Geometry check sheet. Reference: the model listing, model coordinates, mm. Face numbers are marked on the shaded views. Coordinates: 2 decimals unless noted, no trailing zeros. Loops run counter-clockwise (first coordinate to the right, second up) from the corner with the lowest first, then second, coordinate; pieces in that order, holes last.
from build123d import *

# Parameters (mm, degrees)
SKETCH2_R                = 0.85
CUT_EXTRUDE1_DEPTH       = 2.54
BOSS_EXTRUDE1_DEPTH      = 12.7
BOSS_EXTRUDE1_DEPTH_BACK = 2.54
SKETCH3_R                = 1.9
SKETCH4_R                = 0.85
CUT_EXTRUDE2_DEPTH       = 2.794


with BuildPart() as part:
    # Sketch1 → Revolve1 (revolve)
    with BuildSketch(Plane.XY, mode=Mode.PRIVATE) as revolve1_sk:
        Polygon((0, 0), (0, 8.5), (5.21775571, 8.5), (5.21775571, 8), (5.71775571, 8), (5.71775571, 8.5), (11.139308543, 8.5), (11.139308543, 8), (11.639308543, 8), (11.639308543, 8.5), (14.5, 8.5), (14.5, 0), align=None)
    revolve(revolve1_sk.sketch.rotate(Axis((0, 0, 0), (1, 0, 0)), 90), axis=Axis((0, 0, 0), (1, 0, 0)))

    # Sketch2 → Cut-Extrude1 (cut)
    with BuildSketch(Plane.ZY):
        with Locations((-2.641364136, 5.664423669)):
            Circle(SKETCH2_R)
        with Locations((6.226216863, -0.544723392)):
            Circle(SKETCH2_R)
        with Locations((-3.584852727, -5.119700277)):
            Circle(SKETCH2_R)
    extrude(amount=-CUT_EXTRUDE1_DEPTH, mode=Mode.SUBTRACT)

    # Sketch3 → Boss-Extrude1 (add, two sides: drawn at the far end of the back side and taken through both)
    with BuildSketch(Plane(origin=(0, -7.361215932, 4.25), x_dir=(1, 0, 0), z_dir=(0, -0.8660254037844398, 0.499999999999998)).offset(-BOSS_EXTRUDE1_DEPTH_BACK)):
        with Locations(Location((2.694505782, 0, 0), (0, 0, 270))):
            Circle(SKETCH3_R)
    extrude(amount=BOSS_EXTRUDE1_DEPTH + BOSS_EXTRUDE1_DEPTH_BACK)

    # Sketch4 → Cut-Extrude2 (cut)
    with BuildSketch(Plane(origin=(14.5, 0, 0), x_dir=(0, 0, -1), z_dir=(1, 0, 0))):
        with Locations((0, -6.25)):
            Circle(SKETCH4_R)
        with Locations((-5.412658774, 3.125)):
            Circle(SKETCH4_R)
        with Locations((5.412658774, 3.125)):
            Circle(SKETCH4_R)
    extrude(amount=-CUT_EXTRUDE2_DEPTH, mode=Mode.SUBTRACT)


solid = part.part
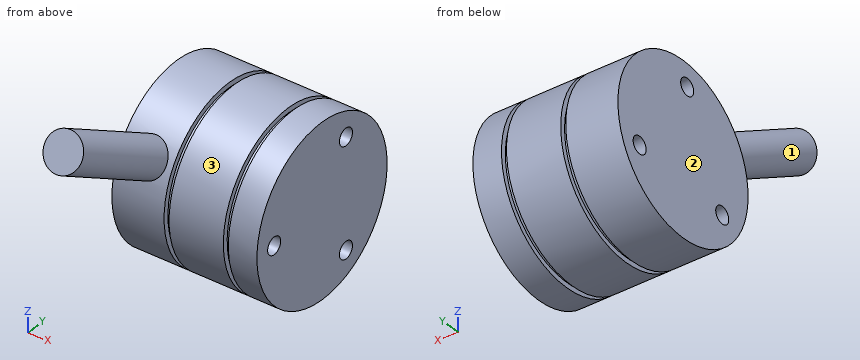
(1) Sectioned sample at A-A on z = 0. Record the cut outline in (x, y), and give its area (3 significant figures).
Findings:
outline: (0, -8.5) - (5.22, -8.5) - (5.22, -8) - (5.72, -8) - (5.72, -8.5) - (11.14, -8.5) - (11.14, -8) - (11.64, -8) - (11.64, -8.5) - (14.5, -8.5) - (14.5, -7.1) - (11.71, -7.1) - (11.71, -5.4) - (14.5, -5.4) - (14.5, 8.5) - (11.64, 8.5) - (11.64, 8) - (11.14, 8) - (11.14, 8.5) - (5.72, 8.5) - (5.72, 8) - (5.22, 8) - (5.22, 8.5) - (0, 8.5) - close
area: 241 mm2
(2) Sectioned sample at B-B on y = 0. Record the cut outline in (x, z), and give its area (3 significant figures).
Findings:
outline: (0, -8.5) - (5.22, -8.5) - (5.22, -8) - (5.72, -8) - (5.72, -8.5) - (11.14, -8.5) - (11.14, -8) - (11.64, -8) - (11.64, -8.5) - (14.5, -8.5) - (14.5, 8.5) - (11.64, 8.5) - (11.64, 8) - (11.14, 8) - (11.14, 8.5) - (5.72, 8.5) - (5.72, 8) - (5.22, 8) - (5.22, 8.5) - (0, 8.5) - (0, 6.88) - (2.54, 6.88) - (2.54, 5.57) - (0, 5.57) - close
area: 242 mm2
(3) Sectioned sample at C-C on x = 6.25. Record the cut outline in (y, z).
Findings:
outline: circle Ø17 at (0, 0)
(4) Gauge pin test, flat ends, axial feed: pin 1 Ø1.5 at (x, y) = (3, 3.5) entering from -Z; pin 2 Ø5 at (x, y) = (1.5, -7) entering from +Z; pin 3 Ø1.4 at (y, z) = (-0.54, 6.23) entering from -X. Record the tip position at first contact, or that the pin passes through.
Findings:
pin 1: stops at z = -8.04
pin 2: stops at z = 7.56
pin 3: stops at x = 2.54
(5) Sectioned sample at D-D on x = 13. Record the cut outline in (y, z) (3 decimals).
Findings:
outline: circle Ø17 at (0, 0); hole circle Ø1.7 at (-6.25, 0); hole circle Ø1.7 at (3.125, -5.413); hole circle Ø1.7 at (3.125, 5.413)
(6) Scan lines: L1, parallel to Y at x = 2.25, z = 6; L2, parallel to Z at x = 2.75, y = 2.75; L3, parallel to Z at x = 1.5, y = 1. Record each from-to range of solid material in increasing order.
Findings:
L1: y = -14.09 to -6.7, -6.02 to -1.36, 0.27 to 6.02
L2: z = -8.04 to 8.04
L3: z = -8.44 to 8.44
(7) Draft check along Y on the marked faces 1, 2 and 3. Enter one of: +Y half, -Y half, draft (parallel to the pull), parting line (faces both ways), or undercut.
Findings:
face 1: undercut
face 2: draft
face 3: parting line
